```python
from build123d import *

# Parameters (mm, degrees)
F2_R     = 0.1
F3_R     = 0.6
F4_DEPTH = 25


with BuildPart() as f1:
    # F0 (on Front) → F1 (revolve)
    with BuildSketch(Plane.XZ):
        with BuildLine():
            Line((2.5, 6), (1.5, 6))
            Line((1.5, 6), (1.5, 3.25))
            ThreePointArc((1.5, 3.25), (3.149178, 2.983027), (4.5, 2))
            Line((4.5, 2), (4.5, -3))
            ThreePointArc((4.5, -3), (3.548227, -3.936809), (2.25, -4.25))
            Line((2.25, -4.25), (2.25, -6))
            Line((2.25, -6), (3.25, -6))
            Line((3.25, -6), (3.25, -5))
            ThreePointArc((3.25, -5), (4.70978, -4.376627), (5.5, -3))
            Line((5.5, -3), (5.5, 2))
            ThreePointArc((5.5, 2), (4.268624, 3.402936), (2.5, 4))
            Line((2.5, 4), (2.5, 6))
        make_face()
    revolve(axis=Axis((0, 0, 2), (0, 0, 1)))

    # F2
    f2_edges = [f1.edges().sort_by_distance(p)[0] for p in [
        (-5.5, 0, 2),
        (-5.5, 0, -3),
    ]]
    fillet(f2_edges, radius=F2_R)

    # F3 (on Right) → F4 (cut)
    with BuildSketch(Plane.YZ):
        with Locations((-2.5, 1)):
            Circle(F3_R)
        with Locations((2.5, 1)):
            Circle(F3_R)
        with BuildLine():
            Line((2, -0.5), (0, -0.5))
            Line((0, -0.5), (0, -2.5))
            ThreePointArc((0, -2.5), (1.310029, -1.810029), (2, -0.5))
        make_face()
        with BuildLine():
            Line((0, -2.5), (0, -0.5))
            Line((0, -0.5), (-2, -0.5))
            ThreePointArc((-2, -0.5), (-1.310029, -1.810029), (0, -2.5))
        make_face()
    extrude(amount=-F4_DEPTH, mode=Mode.SUBTRACT)


solid = f1.part
```
Build history of the part. All positions in model axes, mm. A direction names the side the tool comes from. Round coordinates to 2 decimals unless told otherwise and drop trailing zeros. Write each loop counter-clockwise with the first axis right and the second up, starting at its lowest first coordinate (ties: lowest second). Pieces come first, ordered by that corner, then holes. Notation, with made-up numbers: (-5, 48.25) -> (39, 48.25) arc R13 cw to (39, 61.25) -> close; hole circle Ø9 at (-32.5, 88). An arc over 180 degrees is marked (long way). Put each result on its own line as item: value.
Item 1: Wall check: probe 1 along X at (y, z) = (0, 0.4); probe 2 along Y at (x, z) = (0, 4.3); probe 3 along X at (y, z) = (1.75, 2.5). Give the ranges that are in metal, low to high. Write a range as from..to.
Here are the results:
probe 1: x = -5.5..-4.5, 4.5..5.5
probe 2: y = -2.5..-1.5, 1.5..2.5
probe 3: x = -4.9..-3.57, 3.57..4.9
Item 2: Two-plate mould, pull along X, no slides. Class faces 4 (the face through (-4.2, 3.072, 1.18)), 5 (the face through (4.292, 1.352, -0.535)), 6 (the face through (-0.54, -2.44, 5.01)): pulls with the +X half, pulls with the -X half, needs draft (parallel to the pull), parting line crosses it, or undercut.
Here are the results:
face 4: needs draft
face 5: undercut
face 6: parting line crosses it
Item 3: Flat gauge pins, fed straight in: P1, Ø2, axis at x = -2.5, z = 0, coming from the -Y side; P2, Ø1.9, axis at y = 2.5, z = 1, coming from the -X side; P3, Ø1.5, axis at y = -3, z = 1.5, coming from the -X side. Where does each tip first touch, or does it go through?
Here are the results:
P1: stops at y = -5.29
P2: stops at x = -5.28
P3: stops at x = -5.02
Item 4: Slice it at A-A, the plane z = 1. Give the cut face in (x, y).
Here are the results:
outline: (-5.16, -1.9) -> (-4.08, -1.9) arc R4.5 cw to (-4.08, 1.9) -> (-5.16, 1.9) arc R5.5 ccw to start; (-4.54, -3.1) arc R5.5 ccw (long way) to (-4.54, 3.1) -> (-3.26, 3.1) arc R4.5 cw (long way) to (-3.26, -3.1) -> close
Item 5: Tool access for faces 1 (the face through (-4.2, -2.94, 1.41)), 2 (the face through (-1.5, 0.07, 4.61)), 3 (the face through (-2.579, -1.978, -5.493)): list every direction of +Z, -Z, +X, -X, +Y, -Y with a clear straight run to the whole face (end or side of a thin tool).
Here are the results:
face 1: -X
face 2: +Z, -Z
face 3: -Z
Item 6: Slice it at C-C, the plane y = 1. Count the separate pieces of the cut face and the enclosed holes in it, plus the area to 3 significant figures.
Here are the results:
separate pieces: 3
enclosed holes: 0
area: 29.6 mm^2
Item 7: Slice it at B-B, the plane z = 5.25. Give the cut face in (x, y), plus the area to 3 significant figures.
Here are the results:
outline: circle Ø5 at (0, 0); hole circle Ø3 at (0, 0)
area: 12.6 mm^2
